Read the model definition and answer for the solid it produces. Units are mm, in the model's axes. A direction names the side the tool comes from. Coordinates: 2 decimals unless noted, no trailing zeros. Order: outer loops, then holes, each group sorted by start corner. A loop starts at its lowest first (then second) coordinate and runs counter-clockwise, first axis right, second up. Notation, with made-up numbers: (7, 3.5) -> (44, 3.5) arc R29 cw to (44, 26.5) -> close; hole circle Ø10 at (87, -28.5). An arc over 180 degrees is marked (long way). Answer in a Markdown table with one row per item.
from build123d import *

# Parameters (mm, degrees)
CROQUIS1_R              = 30
SALIENTE_EXTRUIR1_DEPTH = 10.5
CROQUIS2_R              = 24.85
SALIENTE_EXTRUIR2_DEPTH = 1.7
CROQUIS4_R              = 1.5
CORTAR_EXTRUIR1_DEPTH   = 44.706406853
CORTAR_EXTRUIR2_DEPTH   = 10.5
CROQUIS6_R              = 3.15
CORTAR_EXTRUIR3_DEPTH   = 45.145667964


with BuildPart() as part:
    # Croquis1 → Saliente-Extruir1 (new body)
    with BuildSketch(Plane(origin=(0, 0, 0), x_dir=(1, 0, 0), z_dir=(0, 1, 0))):
        with Locations(Location((0, 0, 0), (0, 0, 90))):
            Circle(CROQUIS1_R)
    extrude(amount=SALIENTE_EXTRUIR1_DEPTH)

    # Croquis2 → Saliente-Extruir2 (add)
    with BuildSketch(Plane(origin=(0, 10.5, 0), x_dir=(1, 0, 0), z_dir=(0, 1, 0))):
        with Locations(Location((0, 0, 0), (0, 0, 270))):
            Circle(CROQUIS2_R)
    extrude(amount=SALIENTE_EXTRUIR2_DEPTH)

    # Croquis4 → Cortar-Extruir1 (cut, through all)
    with BuildSketch(Plane(origin=(0, 10.5, 0), x_dir=(1, 0, 0), z_dir=(0, 1, 0))):
        with Locations(Location((-27.5, 0, 0), (0, 0, 270))):
            Circle(CROQUIS4_R)
        with Locations(Location((-17.145969551, 21.500365768, 0), (0, 0, 270))):
            Circle(CROQUIS4_R)
        with Locations(Location((6.119325684, 26.810517585, 0), (0, 0, 270))):
            Circle(CROQUIS4_R)
        with Locations(Location((24.776643867, 11.931802826, 0), (0, 0, 270))):
            Circle(CROQUIS4_R)
        with Locations(Location((24.776643867, -11.931802826, 0), (0, 0, 270))):
            Circle(CROQUIS4_R)
        with Locations(Location((6.119325684, -26.810517585, 0), (0, 0, 270))):
            Circle(CROQUIS4_R)
        with Locations(Location((-17.145969551, -21.500365768, 0), (0, 0, 270))):
            Circle(CROQUIS4_R)
    extrude(amount=-CORTAR_EXTRUIR1_DEPTH, mode=Mode.SUBTRACT)

    # Croquis5 → Cortar-Extruir2 (cut)
    with BuildSketch(Plane.XZ):
        with BuildLine():
            Line((-4.135214626, 9.05), (4.135214626, 9.05))
            ThreePointArc((4.135214626, 9.05), (4.370264873, 9.021983221), (4.592144419, 8.939502762))
            ThreePointArc((4.592144419, 8.939502762), (10.05, 0), (4.592144419, -8.939502762))
            ThreePointArc((4.592144419, -8.939502762), (4.370264873, -9.021983221), (4.135214626, -9.05))
            Line((4.135214626, -9.05), (-4.135214626, -9.05))
            ThreePointArc((-4.135214626, -9.05), (-4.370264873, -9.021983221), (-4.592144419, -8.939502762))
            ThreePointArc((-4.592144419, -8.939502762), (-10.05, 0), (-4.592144419, 8.939502762))
            ThreePointArc((-4.592144419, 8.939502762), (-4.370264873, 9.021983221), (-4.135214626, 9.05))
        make_face()
    extrude(amount=-CORTAR_EXTRUIR2_DEPTH, mode=Mode.SUBTRACT)

    # Croquis6 → Cortar-Extruir3 (cut, through all)
    with BuildSketch(Plane(origin=(0, 12.2, 0), x_dir=(1, 0, 0), z_dir=(0, 1, 0))):
        with Locations(Location((0, 0, 0), (0, 0, 270))):
            Circle(CROQUIS6_R)
    extrude(amount=-CORTAR_EXTRUIR3_DEPTH, mode=Mode.SUBTRACT)


solid = part.part
Q1. The part is cut by section B-B (z = 0). Write down the section's boundary in (x, y).
Outcome:
| item | result |
|---|---|
| outline | (-30, 0) -> (-29, 0) -> (-29, 10.5) -> (-30, 10.5) -> close; (-26, 0) -> (-10.05, 0) -> (-10.05, 10.5) -> (-3.15, 10.5) -> (-3.15, 12.2) -> (-24.85, 12.2) -> (-24.85, 10.5) -> (-26, 10.5) -> close; (3.15, 10.5) -> (10.05, 10.5) -> (10.05, 0) -> (30, 0) -> (30, 10.5) -> (24.85, 10.5) -> (24.85, 12.2) -> (3.15, 12.2) -> close |
Q2. The part is cut by section A-A (x = 0). Write down the section's boundary in (y, z), then the cut area to 3 significant figures.
Outcome:
| item | result |
|---|---|
| outline | (0, -30) -> (10.5, -30) -> (10.5, -24.85) -> (12.2, -24.85) -> (12.2, -3.15) -> (10.5, -3.15) -> (10.5, -9.05) -> (0, -9.05) -> close; (0, 9.05) -> (10.5, 9.05) -> (10.5, 3.15) -> (12.2, 3.15) -> (12.2, 24.85) -> (10.5, 24.85) -> (10.5, 30) -> (0, 30) -> close |
| area | 514 mm² |
Q3. For a pull along X with two mould halves and no side action, classify faces 4 (the face through (23.446, 5.324, -11.24)), 5 (the face through (13, 0, 0)), 6 (the face through (-9.518, 11.338, 22.955)) as pulls with the +X half, pulls with the -X half, needs draft (parallel to the pull), parting line crosses it, or undercut.
Outcome:
| item | result |
|---|---|
| face 4 | undercut |
| face 5 | needs draft |
| face 6 | parting line crosses it |
Q4. Given pin 1 (1 mm diameter, centred on x = -3, y = 7.5, fed in from -Z); pin 2 (5 mm diameter, centred on x = 6.12, z = -26.81, fed in from +Y); pin 3 (1.5 mm diameter, centred on y = 10.5, z = -7, fed in from -X), each flat-ended and moving along its own axis, determine where each tip first touches the part or whether it passes through.
Outcome:
| item | result |
|---|---|
| pin 1 | z = -29.9 |
| pin 2 | y = 10.5 |
| pin 3 | x = -29.34 |
Q5. The part is cut by section C-C (y = 6.25). Give the number of separate pieces and of enclosed holes in the cut face, then the cut area to 3 significant figures.
Outcome:
| item | result |
|---|---|
| separate pieces | 1 |
| enclosed holes | 8 |
| area | 2,470 mm² |
Q6. Consider line 1 (Z direction, x = 6.5, y = 7); line 2 (Z direction, x = 7, y = 2.5); line 3 (Z direction, x = -0.5, y = 4.5). Determine where each line is inside the solid, lowest interval first.
Outcome:
| item | result |
|---|---|
| line 1 | -29.29 to -28.26, -25.36 to -7.67, 7.67 to 25.36, 28.26 to 29.29 |
| line 2 | -29.17 to -28.02, -25.6 to -7.21, 7.21 to 25.6, 28.02 to 29.17 |
| line 3 | -30 to -9.05, 9.05 to 30 |
Q7. The part is cut by section D-D (z = 12). Write down the section's boundary in (x, y), then the cut area to 3 significant figures.
Outcome:
| item | result |
|---|---|
| outline | (-27.5, 0) -> (23.28, 0) -> (23.28, 10.5) -> (21.76, 10.5) -> (21.76, 12.2) -> (-21.76, 12.2) -> (-21.76, 10.5) -> (-27.5, 10.5) -> close; (26.28, 0) -> (27.5, 0) -> (27.5, 10.5) -> (26.28, 10.5) -> close |
| area | 620 mm² |
Q8. For faces 1 (the face through (4, 10.5, 25)), 2 (the face through (4.789, 5.324, 27.503)), 3 (the face through (0, 5, -9.05)), determine the directions among +Z, -Z, +X, -X, +Y, -Y from which every point of the face is accessible in a straight line to the end or side of a thin tool.
Outcome:
| item | result |
|---|---|
| face 1 | +Y |
| face 2 | +Y, -Y |
| face 3 | -Y |
